Can you work these out from the drawing? Everything is in mm from the part's minimum corner. Round coordinates to 2 decimals unless told otherwise and drop trailing zeros. Write each loop counter-clockwise with the first axis right and the second up, starting at its lowest first coordinate (ties: lowest second). Pieces come first, ordered by that corner, then holes. Notation, with made-up numbers: (-27, 81) - (-4, 81) arc R18 cw to (-4, 88) - close; hole circle Ø9 at (-5, 66). An arc over 180 degrees is marked (long way). One line per item, written item: value. Start each with the question number.
Item 1: Imagine slicing it at D-D, the plane x = 138.7. Please give me the cut outline in (y, z), then the cut area to 3 significant figures.
Item 2: Imagine slicing it at C-C, the plane x = 82.5. Please give me the cut outline in (y, z), then the cut area to 3 significant figures.
Item 3: Imagine slicing it at A-A, the plane z = 134. Please give me the cut outline in (x, y), then the cut area to 3 significant figures.
Item 4: If I drill on line 1 (Z direction, x = 89, y = 2.25); line 2 (X direction, y = 2, z = 75); line 3 (Z direction, x = 6.5, y = 1.45), over which ranges is the centre line in solid material (lowest first)?
Item 5: Imagine slicing it at B-B, the plane y = 0.8. Please give me the cut outline in (x, z).
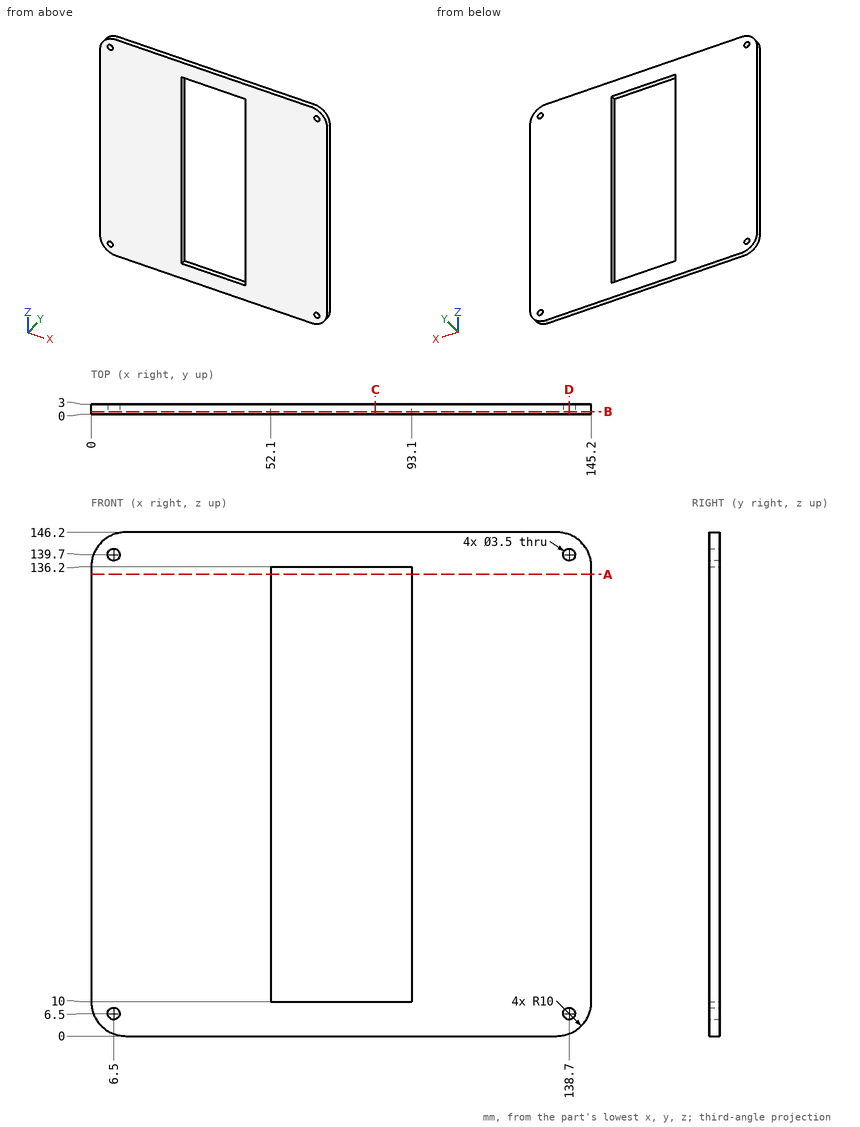
Values follow:
1. outline: (0, 0.63) - (3, 0.63) - (3, 4.75) - (0, 4.75) - close; (0, 8.25) - (3, 8.25) - (3, 137.95) - (0, 137.95) - close; (0, 141.45) - (3, 141.45) - (3, 145.57) - (0, 145.57) - close
1. area: 414 mm^2
2. outline: (0, 0) - (3, 0) - (3, 10) - (0, 10) - close; (0, 136.2) - (3, 136.2) - (3, 146.2) - (0, 146.2) - close
2. area: 60.0 mm^2
3. outline: (0, 0) - (52.1, 0) - (52.1, 3) - (0, 3) - close; (93.1, 0) - (145.2, 0) - (145.2, 3) - (93.1, 3) - close
3. area: 313 mm^2
4. line 1: z = 0 to 10, 136.2 to 146.2
4. line 2: x = 0 to 52.1, 93.1 to 145.2
4. line 3: z = 0.63 to 4.75, 8.25 to 137.95, 141.45 to 145.57
5. outline: (0, 10) arc R10 ccw to (10, 0) - (135.2, 0) arc R10 ccw to (145.2, 10) - (145.2, 136.2) arc R10 ccw to (135.2, 146.2) - (10, 146.2) arc R10 ccw to (0, 136.2) - close; hole circle Ø3.5 at (6.5, 6.5); hole circle Ø3.5 at (6.5, 139.7); hole (52.1, 10) - (93.1, 10) - (93.1, 136.2) - (52.1, 136.2) - close; hole circle Ø3.5 at (138.7, 6.5); hole circle Ø3.5 at (138.7, 139.7)
